Work out the finished part from the listing and answer in its coordinate system (mm). A direction names the side the tool comes from. Round coordinates to 2 decimals unless told otherwise and drop trailing zeros. Answer as CSV lines item,"result". Start each with the question number.
Q1. Section A-A on y = 1.3 is taken. Count the separate pieces of the cut face and the enclosed holes in it, then the cut area to 3 significant figures.
Q2. For faces 1 (the face through (-9.99, 1.01, 76.13)), 2 (the face through (1, 2, 1)), determine the directions among +Z, -Z, +X, -X, +Y, -Y from which every point of the face is accessible in a straight line to the end or side of a thin tool.
Q3. The mould has two halves that part along X. Classify faces 3 (the face through (1, 0, 1)), 4 (the face through (9.8, 1.01, 76.32)), 5 (the face through (0, 1, 61)): +X half, -X half, draft (parallel to the pull), parting line (faces both ways), or undercut.
Q4. Straight lines are drawn through the part: L1, parallel to Z at x = -24, y = 1.6; L2, parallel to X at y = 0.55, z = 10; L3, parallel to X at y = 1.05, z = -100. For each, find the intervals that lie inside material, in ascending order. Write a range as [from, to].
Autodesk Inventor part; units mm, degrees
ref_plane "YZ Plane" through (0, 0, 0) normal (1, 0, 0) x (0, 1, 0)
ref_plane "XZ Plane" through (0, 0, 0) normal (0, 1, 0) x (-1, 0, 0)
ref_plane "XY Plane" through (0, 0, 0) normal (0, 0, 1) x (1, 0, 0)
sketch "スケッチ1" plane through (0, 0, 0) normal (0, 1, 0) x (-1, 0, 0)
  line L0 (-87.5, 105) -> (87.5, 105)
  line L1 (87.5, 105) -> (87.5, -105)
  line L2 (87.5, -105) -> (-87.5, -105)
  line L3 (-87.5, -105) -> (-87.5, 105)
  line L4 (-87.5, 105) -> (87.5, -105) construction
  line L5 (87.5, 105) -> (-87.5, -105) construction
  point P0 (0, 0)
  dimension "d0" = 210
  dimension "d1" = 175
extrude "プレート1" add sketch "スケッチ1" along normal blind 2
sketch "スケッチ5" plane through (0, 2, 0) normal (0, 1, 0) x (1, 0, 0)
  line L0 (-24, -101) -> (34.6, -101)
  line L1 (34.6, -101) -> (34.6, -67)
  line L2 (34.6, -67) -> (-24, -67)
  line L3 (-24, -67) -> (-24, -101)
  line L4 (-24, -101) -> (34.6, -67) construction
  line L5 (34.6, -101) -> (-24, -67) construction
  line L6 (87.5, -105) -> (-87.5, -105)
  point P0 (0, 0)
  point P1 (0, -84)
  point P2 (5.3, -84)
  point P3 (5.3, -84)
  dimension "d31" = 58.6
  dimension "d32" = 24
  dimension "d33" = 34
  dimension "d78" = 4
hole "穴3" at (34.6, 2, 67) at (34.6, 2, 101) at (-24, 2, 67) at (-24, 2, 101) direction (0, -1, 0) diameter 4.3 end through all
sketch "スケッチ6" plane through (0, 2, 0) normal (0, 1, 0) x (1, 0, 0)
  line L0 (-133.9967, -217.2896) -> (133.2896, 49.9967)
  line L1 (133.2896, 49.9967) -> (133.9967, 49.2896)
  line L2 (133.9967, 49.2896) -> (-133.2896, -217.9967)
  line L3 (-133.2896, -217.9967) -> (-133.9967, -217.2896)
  line L4 (-133.9967, -217.2896) -> (133.9967, 49.2896) construction
  line L5 (133.2896, 49.9967) -> (-133.2896, -217.9967) construction
  line L6 (133.9967, -217.2896) -> (-133.2896, 49.9967)
  line L7 (-133.2896, 49.9967) -> (-133.9967, 49.2896)
  line L8 (-133.9967, 49.2896) -> (133.2896, -217.9967)
  line L9 (133.2896, -217.9967) -> (133.9967, -217.2896)
  line L10 (133.9967, -217.2896) -> (-133.9967, 49.2896) construction
  line L11 (-133.2896, 49.9967) -> (133.2896, -217.9967) construction
  line L12 (-2.4749, -82.2322) -> (-1.7678, -81.5251)
  circle A0 centre (0, -84) radius 22
  line L13 (2.4749, -82.2322) -> (1.7678, -81.5251)
  circle A1 centre (0, -84) radius 3
  line L14 (-87.5, -105) -> (-87.5, 105)
  line L15 (87.5, 105) -> (87.5, -105)
  line L16 (122.5, 0) -> (-122.5, 0)
  point P0 (0, 0)
  point P1 (0, -84)
  point P2 (-2.1213, -81.8787)
  point P3 (2.1213, -81.8787)
  point P4 (15.9059, -68.8012)
  point P5 (-15.9059, -68.8012)
  dimension "d54" = 1
  dimension "d55" = 1
  dimension "d57" = 44
  dimension "d59" = 3
  dimension "d60" = 3
  dimension "d65" = 186
  dimension "d66" = 186
  dimension "d79" = 45
  dimension "d80" = 45
extrude "押し出し2" cut sketch "スケッチ6" against normal blind 10 contours A0 L6 L12 L8 | A0 L0 A1 L6 | L12 L6 A1 | A0 L2 L13 L0 | L0 L13 A1
sketch "スケッチ7" plane through (0, 2, 0) normal (0, 1, 0) x (1, 0, 0)
  line L0 (-82.5, -100) -> (82.5, -100)
  line L1 (82.5, -100) -> (82.5, 100)
  line L2 (82.5, 100) -> (-82.5, 100)
  line L3 (-82.5, 100) -> (-82.5, -100)
  line L4 (-82.5, -100) -> (82.5, 100) construction
  line L5 (82.5, -100) -> (-82.5, 100) construction
  line L6 (-87.5, -105) -> (-87.5, 105)
  line L7 (87.5, -105) -> (-87.5, -105)
  point P0 (0, 0)
  point P1 (-82.5, -45)
  point P2 (-82.5, -10)
  point P3 (82.5, -45)
  point P4 (82.5, -10)
  dimension "d45" = 5
  dimension "d46" = 5
  dimension "d67" = 55
  dimension "d68" = 35
  dimension "d69" = 55
  dimension "d70" = 35
hole "穴4" at (-82.5, 2, -100) at (82.5, 2, -100) at (-82.5, 2, 100) at (82.5, 2, 100) direction (0, -1, 0) diameter 3.2 end through all
sketch "スケッチ8" plane through (0, 2, 0) normal (0, 1, 0) x (1, 0, 0)
  line L0 (15.9059, -68.8012) -> (2.4749, -82.2322)
  line L1 (-2.1213, -81.8787) -> (-2.4749, -82.2322)
  arc A0 (2.1213, -81.8787) -> (-2.1213, -81.8787) centre (0, -84) ccw
  line L2 (2.4749, -82.2322) -> (2.1213, -81.8787)
  line L3 (-2.4749, -82.2322) -> (-15.9059, -68.8012)
  arc A1 (15.9059, -68.8012) -> (-15.9059, -68.8012) centre (0, -84) ccw
  line L4 (2.4749, -83.6464) -> (17.2895, -68.8318)
  arc A2 (17.2895, -68.8318) -> (-17.2895, -68.8318) centre (0, -84) ccw
  line L5 (-17.2895, -68.8318) -> (-2.4749, -83.6464)
  line L6 (-2.4749, -83.6464) -> (-1.4142, -82.5858)
  arc A3 (1.4142, -82.5858) -> (-1.4142, -82.5858) centre (0, -84) ccw
  line L7 (1.4142, -82.5858) -> (2.4749, -83.6464)
  point P0 (0, 0)
  dimension "d61" = 1
extrude "押し出し3" cut sketch "スケッチ8" against normal blind 10 contours L0 L2 A0 L1 L3 A1 | L7 A3 L6 L5 A2 L4
fillet "コーナーR1" radius 1 4 edges at (-2.4749, 1, 83.6464) (2.4749, 1, 83.6464) (-17.2895, 1, 68.8318) (17.2895, 1, 68.8318)
hole "穴5" at (-82.5, 2, 45) at (-82.5, 2, 10) at (82.5, 2, 45) at (82.5, 2, 10) direction (0, -1, 0) diameter 3.4 end through all
equation "\"d40\" = Thickness"
equation "\"d60\" = d59"
equation "\"d66\" = d65"
equation "\"d76\" = Thickness"
equation "\"d2\" = Thickness"
equation "\"BendRadius\" = Thickness"
equation "\"BendReliefWidth\" = Thickness"
equation "\"BendReliefDepth\" = 0.5 * Thickness"
equation "\"CornerReliefSize\" = 4 * Thickness"
equation "\"MinimumRemnant\" = 2 * Thickness"
equation "\"TransitionRadius\" = BendRadius"
equation "\"JacobiRadiusSize\" = BendRadius"
equation "\"GapSize\" = Thickness"
properties part number "s_carbon_plate1" material "CFRP"
Findings:
1,separate pieces,"1"
1,enclosed holes,"13"
1,area,"36,100 mm^2"
2,face 1,"+Y, -Y"
2,face 2,"+Z, -Z, +X, -X, +Y"
3,face 3,"draft"
3,face 4,"undercut"
3,face 5,"undercut"
4,L1,"z = [-105, 64.85], [69.15, 98.85], [103.15, 105]"
4,L2,"x = [-87.5, -84.2], [-80.8, 80.8], [84.2, 87.5]"
4,L3,"x = [-87.5, -84.1], [-80.9, 80.9], [84.1, 87.5]"
